```python
from build123d import *

# Parameters (mm, degrees)
F0_W     = 94
F0_H     = 12
F1_DEPTH = 2
F3_DEPTH = 5
F4_T     = -2
F5_SIZE  = 5
F6_R     = 1.5
F7_DEPTH = 25
F8_R     = 1.5
F9_DEPTH = 25


with BuildPart() as f1:
    # F0 (on Top) → F1 (new body)
    with BuildSketch(Plane.XY):
        with Locations((-47, -6)):
            Rectangle(F0_W, F0_H)
    extrude(amount=F1_DEPTH)

    # F2 (on face) → F3 (join)
    with BuildSketch(Plane.XY.offset(2)):
        with BuildLine():
            ThreePointArc((-47, -12), (-42.7573593129, -10.2426406871), (-41, -6))
            ThreePointArc((-41, -6), (-42.7573593129, -1.7573593129), (-47, 0))
            ThreePointArc((-47, 0), (-53, -6), (-47, -12))
        make_face()
    extrude(amount=F3_DEPTH)

    # F4
    f4_openings = [f1.faces().sort_by_distance(p)[0] for p in [
        (-47, -6, 7),
    ]]
    offset(amount=F4_T, openings=f4_openings, kind=Kind.INTERSECTION)

    # F5
    f5_edges = [f1.edges().sort_by_distance(p)[0] for p in [
        (-94, -12, 1),
        (-94, 0, 1),
        (0, 0, 1),
        (0, -12, 1),
    ]]
    chamfer(f5_edges, length=F5_SIZE)

    # F6 (on face) → F7 (cut)
    with BuildSketch(Plane.XY.offset(2)):
        with Locations((-47, -6)):
            Circle(F6_R)
    extrude(amount=-F7_DEPTH, mode=Mode.SUBTRACT)

    # F8 (on face) → F9 (cut)
    with BuildSketch(Plane.XY.offset(2)):
        with Locations((-8, -6)):
            Circle(F8_R)
        with Locations((-86, -6)):
            Circle(F8_R)
    extrude(amount=-F9_DEPTH, mode=Mode.SUBTRACT)


solid = f1.part
```
Model file for the job. Use its own axes, mm. A direction names the side the tool comes from. Give positions to 0.01 mm unless a question says otherwise; leave off trailing zeros. Write each loop counter-clockwise with the first axis right and the second up, starting at its lowest first coordinate (ties: lowest second). Pieces come first, ordered by that corner, then holes. Notation, with made-up numbers: (75, -16.5) -> (79, -16.5) arc R17 cw to (79, -6.5) -> close; hole circle Ø3 at (-33.75, 60.5). An arc over 180 degrees is marked (long way). Use CSV: the item, a comma, the result in double quotes. Start each with the question number.
1) Pin check, flat tips, straight feed: P1, Ø1, axis at x = -30.5, y = -3, coming from the +Z side; P2, Ø1, axis at y = -7, z = 5.5, coming from the +X side. Stop position of each tip, or through.
2) Two-plate mould, pull along Y, no slides. Class faces 1 (the cylindrical face through (-84.57, -5.55, 1.01)), 2 (the flat face through (-48, 0, 1)), 3 (the cylindrical face through (-9.5, -5.93, 1.01)), 4 (the flat face through (0, -6, 1)): released by +Y, released by -Y, zero draft, split by the parting line, or undercut.
3) Cut at B-B on z = 1. List the corners of the cut face in (x, y).
4) Drill centre lines: L1, parallel to Y at x = -8, z = 1.55; L2, parallel to Z at x = -6.5, y = -11.25; L3, parallel to X at y = -5.5, z = 3.75. Where is each one in solid material? Low to high.
5) Tool access for faces 5 (the cylindrical face through (-48.5, -5.93, 1.01)), 6 (the flat face through (-47, -8, 2)): list every direction of +Z, -Z, +X, -X, +Y, -Y with a clear straight run to the whole face (end or side of a thin tool).
6) Cut at A-A on x = -86. List the corners of the cut face in (y, z), plus the area to 3 significant figures.
7) Cut at C-C on z = 5.75. List the corners of the cut face in (x, y).
8) Cut at D-D on y = -9. List the corners of the cut face in (x, z).
Final values:
1,P1,"stops at z = 2"
1,P2,"stops at x = -41.02"
2,face 1,"undercut"
2,face 2,"released by +Y"
2,face 3,"undercut"
2,face 4,"zero draft"
3,outline,"(-94, -7) -> (-89, -12) -> (-5, -12) -> (0, -7) -> (0, -5) -> (-5, 0) -> (-89, 0) -> (-94, -5) -> close; hole circle Ø3 at (-86, -6); hole circle Ø3 at (-47, -6); hole circle Ø3 at (-8, -6)"
4,L1,"y = -12 to -7.5, -4.5 to 0"
4,L2,"z = 0 to 2"
4,L3,"x = -52.98 to -50.97, -43.03 to -41.02"
5,face 5,"+Z, -Z"
5,face 6,"+Z"
6,outline,"(-12, 0) -> (-7.5, 0) -> (-7.5, 2) -> (-12, 2) -> close; (-4.5, 0) -> (0, 0) -> (0, 2) -> (-4.5, 2) -> close"
6,area,"18.0 mm2"
7,outline,"circle Ø12 at (-47, -6); hole circle Ø8 at (-47, -6)"
8,outline,"(-92, 0) -> (-2, 0) -> (-2, 2) -> (-41.8, 2) -> (-41.8, 7) -> (-44.35, 7) -> (-44.35, 2) -> (-49.65, 2) -> (-49.65, 7) -> (-52.2, 7) -> (-52.2, 2) -> (-92, 2) -> close"
